Read the model definition and answer for the solid it produces. Units are mm, in the model's axes. A direction names the side the tool comes from. Coordinates: 2 decimals unless noted, no trailing zeros. Write each loop counter-clockwise with the first axis right and the second up, starting at its lowest first coordinate (ties: lowest second). Pieces come first, ordered by that corner, then holes. Notation, with made-up numbers: (63.25, 56.5) -> (98.25, 56.5) arc R22 cw to (98.25, 66.5) -> close; hole circle Ø4 at (59.5, 10.25). An arc over 180 degrees is marked (long way). Answer as a JSON object with one key per item and string values. Group by question number.
(1) Straight lines are drawn through the part: L1, parallel to Z at x = -9.25, y = -1.35; L2, parallel to Z at x = -6.5, y = 1.65; L3, parallel to X at y = 0.6, z = 29.5. For each, find the intervals that lie inside material, in ascending order.
(2) Find section C-C (x = 0). Give the vertices of the cut face in (y, z), then the cut area to 3 significant figures.
(3) Find section D-D (z = 30). Give the vertices of the cut face in (x, y), then the cut area to 3 significant figures.
(4) Flat-ended cylindrical pins translate along their axes: P1, Ø2, axis at x = -3.5, y = -0.5, coming from the +Z side; P2, Ø2, axis at y = 0.5, z = 31.5, coming from the +X side. Find the tip coordinate at first contact, or state that the pin passes through.
(5) Find section A-A (y = -0.1). Give the vertices of the cut face in (x, z).
(6) Which of the six approach directions +Z, -Z, +X, -X, +Y, -Y give full straight-line access (tool end or side, diameter ignored) to faces 1 (the face through (0, -2, 17)), 2 (the face through (-11.95, 0.03, 24)), 3 (the face through (-3, 0, 27)), 4 (the face through (-13, 0, 31))?
(7) Find section B-B (x = -10). Give the vertices of the cut face in (y, z), then the cut area to 3 significant figures.
(8) For a pull along Z with two mould halves and no side action, classify faces 5 (the face through (-6, 0, -2)), 6 (the face through (-6, 0, 23)), 7 (the face through (-11, 0, 36)), 8 (the face through (-13.5, 0, 0)) as +Z half, -Z half, draft (parallel to the pull), parting line (faces both ways), or undercut.
from build123d import *

# Parameters (mm, degrees)
F2_W = 4
F2_H = 4
F4_R = 3.5
F5_R = 1


with BuildPart() as f3:
    # F3: sweep along a path in F0
    with BuildLine(Plane.XZ) as f3_path:
        Line((-13.5, 0), (0, 0))
        Line((0, 0), (0, 25))
        Line((0, 25), (-11, 25))
        Line((-11, 25), (-11, 36))
    # F2 (on line) → F3 (sweep)
    with BuildSketch(Plane(origin=(-13.5, 0, 0), x_dir=(0, -1, 0), z_dir=(-1, 0, 0))):
        Rectangle(F2_W, F2_H)
    sweep(path=f3_path.line, transition=Transition.RIGHT)

    # F4
    f4_edges = [f3.edges().sort_by_distance(p)[0] for p in [
        (-13, 0, 23),
    ]]
    fillet(f4_edges, radius=F4_R)

    # F5
    f5_edges = [f3.edges().sort_by_distance(p)[0] for p in [
        (-9, 0, 27),
        (-2, 0, 2),
    ]]
    fillet(f5_edges, radius=F5_R)


solid = f3.part
Results below:
{
 "1": {"L1": "z = -2 to 2, 23 to 36", "L2": "z = -2 to 2, 23 to 27", "L3": "x = -13 to -9"},
 "2": {"outline": "(-2, -2) -> (2, -2) -> (2, 27) -> (-2, 27) -> close", "area": "116 mm2"},
 "3": {"outline": "(-13, -2) -> (-9, -2) -> (-9, 2) -> (-13, 2) -> close", "area": "16.0 mm2"},
 "4": {"P1": "stops at z = 27", "P2": "stops at x = -9"},
 "5": {"outline": "(-13.5, -2) -> (2, -2) -> (2, 27) -> (-8, 27) arc R1 cw to (-9, 28) -> (-9, 36) -> (-13, 36) -> (-13, 26.5) arc R3.5 ccw to (-9.5, 23) -> (-2, 23) -> (-2, 3) arc R1 cw to (-3, 2) -> (-13.5, 2) -> close"},
 "6": {"face 1": "+Z, -Z, +X, -X, -Y", "face 2": "-X, +Y, -Y", "face 3": "+Z, +X, +Y, -Y", "face 4": "+Z, -X, +Y, -Y"},
 "7": {"outline": "(-2, -2) -> (2, -2) -> (2, 2) -> (-2, 2) -> close; (-2, 23.04) -> (2, 23.04) -> (2, 36) -> (-2, 36) -> close", "area": "67.9 mm2"},
 "8": {"face 5": "-Z half", "face 6": "undercut", "face 7": "+Z half", "face 8": "draft"}
}
